Verification items for the finished model (mm, model axes). A direction names the side the tool comes from. Coordinates: 2 decimals unless noted, no trailing zeros. Order: outer loops, then holes, each group sorted by start corner. A loop starts at its lowest first (then second) coordinate and runs counter-clockwise, first axis right, second up. Notation, with made-up numbers: (34, 70) - (87, 70) arc R18 ccw to (87, 79) - close; hole circle Ø8 at (-31, 27.25). An arc over 180 degrees is marked (long way). One line per question, with ' | ' between items. Start each with the question number.
from build123d import *

# Parameters (mm, degrees)
F2_W         = 3.15
F2_H         = 8
F4_W         = 5.5
F4_H         = 19.5
F5_DEPTH     = 11.5
F6_R         = 2.5
F7_DEPTH     = 5.5
F8_T1_DEPTH  = 1.575
F8_T6_DEPTH  = 8
F8_T12_DEPTH = 18
F8_T17_DEPTH = 11.575
F9_R         = 0.9
F10_DEPTH    = 3.15


# Not quite as in the source:
# - a fillet or chamfer that OpenCascade refuses, or shapes differently, is made with other operations: its cross-section is extruded or revolved along the edge and cut away or added


with BuildPart() as f3:
    # F3: sweep along a path in F1
    with BuildLine(Plane.YZ) as f3_path:
        Line((0, 0), (-160, 0))
        ThreePointArc((-160, 0), (-177.6776695297, -7.3223304703), (-185, -25))
        Line((-185, -25), (-185, -80))
    # F2 (on Front) → F3 (sweep)
    with BuildSketch(Plane.XZ):
        Rectangle(F2_W, F2_H)
    sweep(path=f3_path.line)

    # F4 (on face) → F5 (join)
    with BuildSketch(Plane(origin=(0, 0, -80), x_dir=(1, 0, 0), z_dir=(0, 0, -1))):
        with Locations((2.75, 179.25)):
            Rectangle(F4_W, F4_H)
    extrude(amount=-F5_DEPTH)

    # F6 (on face) → F7 (cut, through all)
    with BuildSketch(Plane.YZ.offset(5.5)):
        with Locations((-175.25, -74.25)):
            Circle(F6_R)
    extrude(amount=-F7_DEPTH, mode=Mode.SUBTRACT)

    # F8: fillet of radius 4 on 2 edges, made by hand

    # F8_s2 → F8_t1 (join)
    with BuildSketch(Plane.YZ):
        with BuildLine():
            ThreePointArc((-181, -64.5), (-179.8284271247, -67.3284271247), (-177, -68.5))
            Line((-177, -68.5), (-181, -68.5))
            Line((-181, -68.5), (-181, -64.5))
        make_face()
    extrude(amount=F8_T1_DEPTH)


with BuildPart() as f8_tool4:
    # F8_s5 → F8_t6 (new body)
    with BuildSketch(Plane.XZ.offset(189)):
        with BuildLine():
            ThreePointArc((1.575, -64.5), (2.7465728753, -67.3284271247), (5.575, -68.5))
            Line((5.575, -68.5), (1.575, -68.5))
            Line((1.575, -68.5), (1.575, -64.5))
        make_face()
    extrude(amount=-F8_T6_DEPTH)

    split(bisect_by=Plane.YZ.offset(5.5), keep=Keep.BOTTOM)


with BuildPart() as f3_1:
    add(f3.part)

    # F8_t3: union F8_tool4
    add(f8_tool4.part)


with BuildPart() as f8_tool10:
    # F8_s11 → F8_t12 (new body)
    with BuildSketch(Plane.XZ.offset(189)):
        with BuildLine():
            ThreePointArc((1.575, -64.5), (2.7465728753, -67.3284271247), (5.575, -68.5))
            Line((5.575, -68.5), (1.575, -68.5))
            Line((1.575, -68.5), (1.575, -64.5))
        make_face()
    extrude(amount=-F8_T12_DEPTH)

    split(bisect_by=Plane.XZ.offset(181), keep=Keep.BOTTOM)

    split(bisect_by=Plane.YZ.offset(5.5), keep=Keep.BOTTOM)


with BuildPart() as f8_tool15:
    # F8_s16 → F8_t17 (new body)
    with BuildSketch(Plane.YZ.offset(11.575)):
        with BuildLine():
            ThreePointArc((-181, -64.5), (-179.8284271247, -67.3284271247), (-177, -68.5))
            Line((-177, -68.5), (-181, -68.5))
            Line((-181, -68.5), (-181, -64.5))
        make_face()
    extrude(amount=-F8_T17_DEPTH)

    split(bisect_by=Plane.YZ.offset(1.575), keep=Keep.TOP)

    split(bisect_by=Plane.YZ.offset(5.5), keep=Keep.BOTTOM)


with BuildPart() as f8_tool10_1:
    add(f8_tool10.part)

    # F8_t20: intersect F8_tool15
    add(f8_tool15.part, mode=Mode.INTERSECT)


with BuildPart() as f3_2:
    add(f3_1.part)

    # F8_t8: union F8_tool10
    add(f8_tool10_1.part)

    # F9 (on face) → F10 (cut, through all)
    with BuildSketch(Plane.YZ.offset(1.575)):
        with Locations((-5, 0)):
            Circle(F9_R)
    extrude(amount=-F10_DEPTH, mode=Mode.SUBTRACT)


solid = f3_2.part
Item 1: Section check D-D (y = -122). Record the cut outline in (x, z) (3 decimals).
Item 2: Gauge pin test, flat ends, axial feed: pin 1 (1.5 mm diameter, centred on x = 3, y = -40.5, fed in from +Z); pin 2 (6 mm diameter, centred on y = -175.5, z = -71.5, fed in from -X); pin 3 (2.5 mm diameter, centred on x = 0, y = -49, fed in from -Z); pin 4 (0.9 mm diameter, centred on x = 0, z = -66, fed in from +Y). Record the tip position at first contact, or that the pin passes through.
Item 3: Thickness scan on probe 1 along Z at (x, y) = (3.6, -175.25); probe 2 along Z at (x, y) = (-0.2, -5); probe 3 along Z at (x, y) = (0.5, -122). Record the ranges inside material, lowest first. Write a range as from..to.
Item 4: Section check C-C (y = -175.25). Record the cut outline in (x, z) (3 decimals).
Item 5: Section check A-A (z = -74.25). Record the cut outline in (x, y) (3 decimals).
Item 6: Set-up check for faces 1 (the cylindrical face through (1.57, -179.33, -67.75)), 2 (the flat face through (0, -181, -47)), 3 (the flat face through (0, -178, -74)): record each of +Z, -Z, +X, -X, +Y, -Y from which the full face is reachable in a straight line by a thin tool's end or side.
Item 7: Mould release check, pull along Z, two halves, no side actions. Record for faces 4 (the flat face through (1.575, -108, -2)), 5 (the cylindrical face through (2.69, -184.45, -67.27)), 6 (the cylindrical face through (2.79, -172.94, -75.21)): +Z half, -Z half, draft (parallel to the pull), parting line (faces both ways), or undercut.
Item 8: Section check B-B (x = 3). Record the cut outline in (y, z) (3 decimals), then the cut area to 3 significant figures.
Completed:
1) outline: (-1.575, -4) - (1.575, -4) - (1.575, 4) - (-1.575, 4) - close
2) pin 1: passes through | pin 2: stops at x = 0 | pin 3: stops at z = -4 | pin 4: stops at y = -180.49
3) probe 1: z = -80..-76.75, -71.75..-68.5 | probe 2: z = -4..-0.9, 0.9..4 | probe 3: z = -4..4
4) outline: (-1.575, -10.563) - (1.575, -10.563) - (1.575, -0.333) - (-1.575, -0.333) - close; (0, -80) - (5.5, -80) - (5.5, -76.75) - (0, -76.75) - close; (0, -71.75) - (5.5, -71.75) - (5.5, -68.5) - (0, -68.5) - close
5) outline: (-1.575, -189) - (5.5, -189) - (5.5, -177.75) - (0, -177.75) - (0, -181) - (-1.575, -181) - close; (0, -172.75) - (5.5, -172.75) - (5.5, -169.5) - (0, -169.5) - close
6) face 1: +X, -X, +Y | face 2: -X, +Y | face 3: -Z, -X, +Y
7) face 4: draft | face 5: +Z half | face 6: undercut
8) outline: (-189, -80) - (-169.5, -80) - (-169.5, -68.5) - (-177, -68.5) arc R4 cw to (-179.575, -67.561) - (-189, -67.561) - close; hole circle Ø5 at (-175.25, -74.25) | area: 214 mm^2
